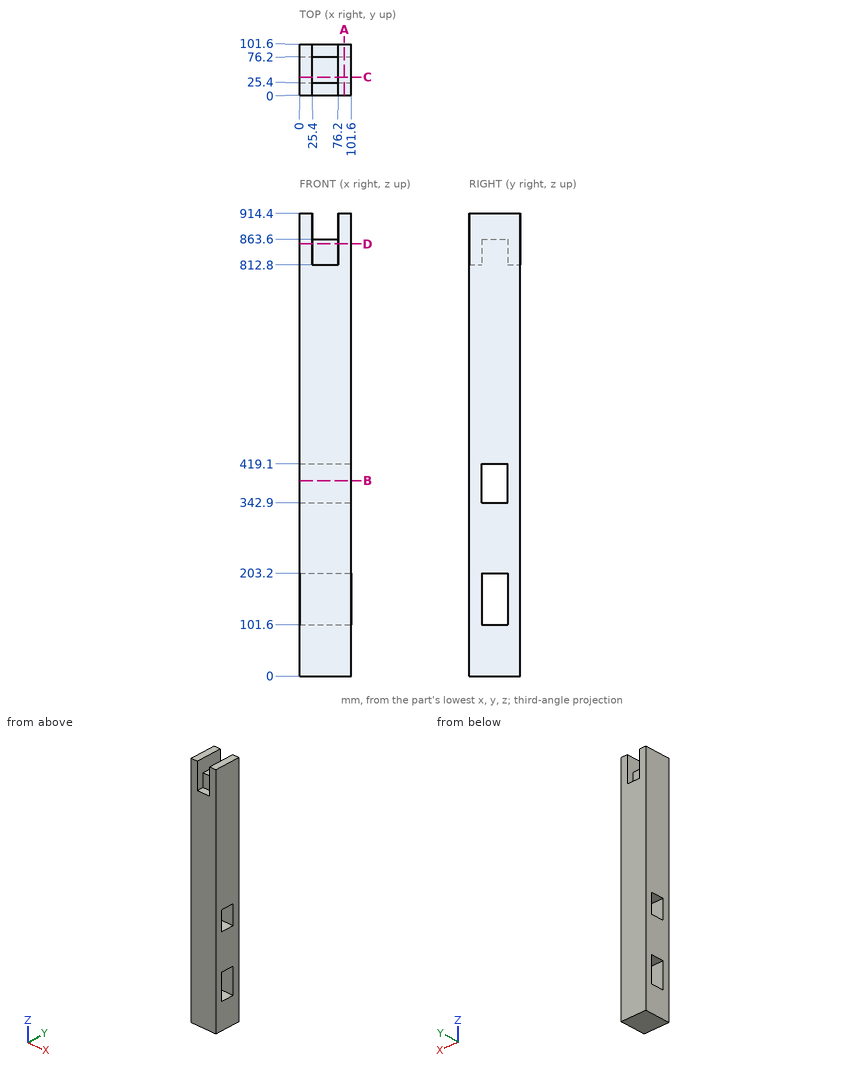
Job drawing, mm, ordinate dimensions from the low corner. One solid piece. Give positions to 0.01 mm unless a question says otherwise; leave off trailing zeros. Loops run counter-clockwise (first coordinate to the right, second up) from the corner with the lowest first, then second, coordinate; pieces in that order, holes last. Notation, with made-up numbers: (50.25, 67.5) - (88.25, 67.5) arc R13 ccw to (88.25, 83.5) - close; hole circle Ø4 at (64.25, 59). An arc over 180 degrees is marked (long way). Use one line per item in the form item = value.
(1) Cut at D-D (z = 854). Give the cut face in (x, y).
Determined:
outline = (0, 0) - (25.4, 0) - (25.4, 25.4) - (76.2, 25.4) - (76.2, 0) - (101.6, 0) - (101.6, 101.6) - (76.2, 101.6) - (76.2, 76.2) - (25.4, 76.2) - (25.4, 101.6) - (0, 101.6) - close
(2) Drill centre lines: L1, parallel to Z at x = 88.5, y = 56.5; L2, parallel to Z at x = 26.5, y = 26; L3, parallel to Y at x = 85, z = 151. Where is each one in solid material? Low to high.
Determined:
L1 = 0 to 101.6, 203.2 to 342.9, 419.1 to 914.4
L2 = 0 to 101.6, 203.2 to 342.9, 419.1 to 863.6
L3 = 0 to 25.4, 76.2 to 101.6
(3) Cut at A-A (x = 88.5). Give the cut face in (y, z), then the cut area to 3 significant figures.
Determined:
outline = (0, 0) - (101.6, 0) - (101.6, 914.4) - (0, 914.4) - close; hole (25.4, 101.6) - (76.2, 101.6) - (76.2, 203.2) - (25.4, 203.2) - close; hole (25.4, 342.9) - (76.2, 342.9) - (76.2, 419.1) - (25.4, 419.1) - close
area = 83,900 mm^2
(4) Cut at B-B (z = 386). Give the cut face in (x, y), then the cut area to 3 significant figures.
Determined:
outline = (0, 0) - (101.6, 0) - (101.6, 25.4) - (0, 25.4) - close; (0, 76.2) - (101.6, 76.2) - (101.6, 101.6) - (0, 101.6) - close
area = 5,160 mm^2
(5) Drop flat-ended pins along their axis: P1, Ø2, axis at x = 64.5, y = 16.5, coming from the +Z side; P2, Ø15, axis at x = 47.5, z = 849.5, coming from the -Y side. Give the stop position or say it passes through.
Determined:
P1 = 812.8
P2 = 25.4
(6) Cut at C-C (y = 36). Give the cut face in (x, z), then the cut area to 3 significant figures.
Determined:
outline = (0, 0) - (101.6, 0) - (101.6, 101.6) - (0, 101.6) - close; (0, 203.2) - (101.6, 203.2) - (101.6, 342.9) - (0, 342.9) - close; (0, 419.1) - (101.6, 419.1) - (101.6, 914.4) - (76.2, 914.4) - (76.2, 863.6) - (25.4, 863.6) - (25.4, 914.4) - (0, 914.4) - close
area = 72,300 mm^2
